Can you work these out from the drawing? Everything is in mm from the part's minimum corner. A direction names the side the tool comes from. Round coordinates to 2 decimals unless told otherwise and drop trailing zeros. Write each loop counter-clockwise with the first axis right and the second up, starting at its lowest first coordinate (ties: lowest second). Pieces come first, ordered by that corner, then holes. Notation, with made-up numbers: (80, 30.25) - (106, 30.25) arc R28 cw to (106, 66.25) - close; hole circle Ø1 at (8.25, -20.5). An arc over 180 degrees is marked (long way). One line per item, written item: value. Start each with the question number.
Item 1: For the marked faces 1, 2 and 3, which set-ups out of +Z, -Z, +X, -X, +Y, -Y let a thin tool reach every point of the face, with its end or its side?
Item 2: For P1, Ø4, axis at x = 20, z = 34.5, coming from the -Y side; P2, Ø5, axis at x = 35, z = 31.5, coming from the +Y side; P3, Ø15, axis at y = 23, z = 48.5, coming from the -X side, each with a flat end and sliding along its axis, tell me the tip position at first contact or that it passes through.
Item 3: If I drill on line 1 (Y direction, x = 25, z = 19.25); line 2 (X direction, y = 19, z = 57.5), over which ranges is the centre line in solid material (lowest first)?
Item 4: Imagine slicing it at D-D, the plane z = 35. Please give me the cut outline in (x, y).
Item 5: Imagine slicing it at C-C, the plane z = 10.5. Please give me the cut outline in (x, y), then the cut area to 3 significant figures.
Item 6: Imagine slicing it at A-A, the plane x = 25. Please give me the cut outline in (y, z), then the cut area to 3 significant figures.
Item 7: Thinking about a two-plate mould opening in X: for the marked faces 4, 5 and 6, which applies, released by +X, released by -X, zero draft, split by the parting line, or undercut?
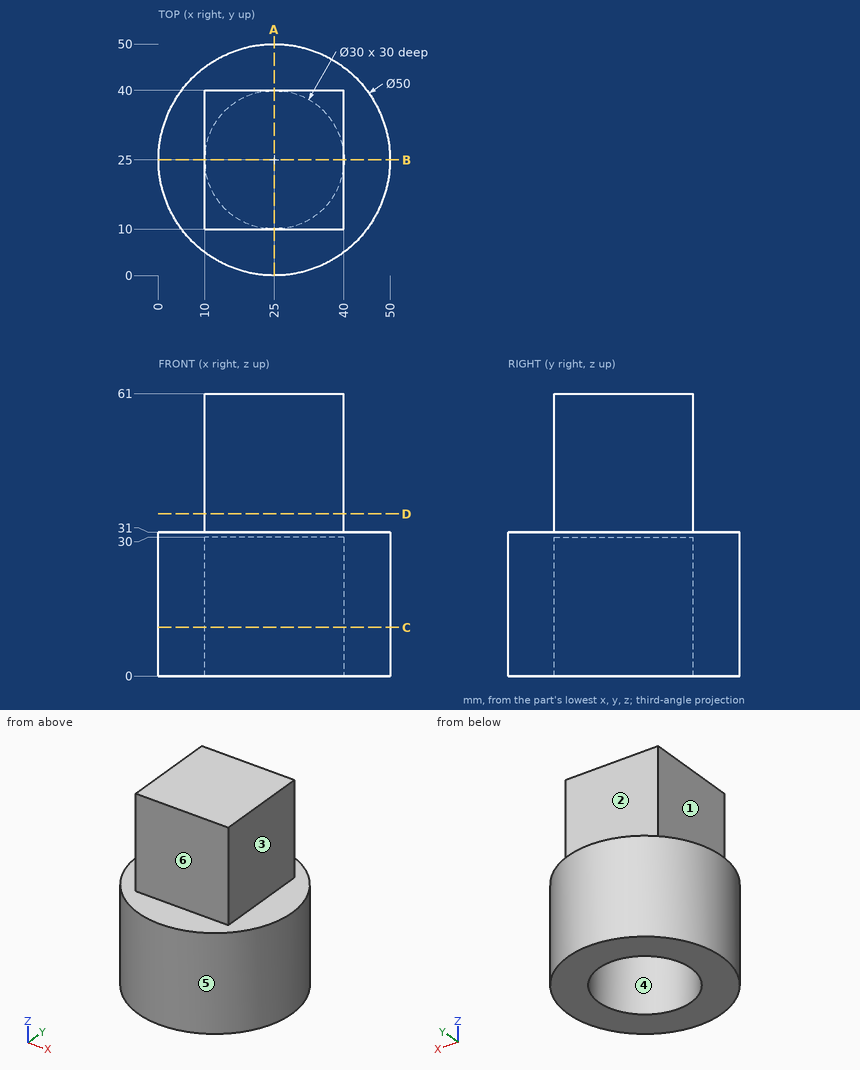
Values follow:
1. face 1: +Z, -X, +Y, -Y
1. face 2: +Z, +X, -X, +Y
1. face 3: +Z, +X, +Y, -Y
2. P1: stops at y = 10
2. P2: stops at y = 48.83
2. P3: stops at x = 10
3. line 1: y = 0 to 10, 40 to 50
3. line 2: x = 10 to 40
4. outline: (10, 10) - (40, 10) - (40, 40) - (10, 40) - close
5. outline: circle Ø50 at (25, 25); hole circle Ø30 at (25, 25)
5. area: 1,260 mm^2
6. outline: (0, 0) - (10, 0) - (10, 30) - (40, 30) - (40, 0) - (50, 0) - (50, 31) - (40, 31) - (40, 61) - (10, 61) - (10, 31) - (0, 31) - close
6. area: 1,550 mm^2
7. face 4: undercut
7. face 5: split by the parting line
7. face 6: zero draft
